Build history of the part. All positions in model axes, mm. A direction names the side the tool comes from. Give positions to 0.01 mm unless a question says otherwise; leave off trailing zeros. Loops run counter-clockwise (first coordinate to the right, second up) from the corner with the lowest first, then second, coordinate; pieces in that order, holes last. Notation, with made-up numbers: (0.25, 17.25) -> (46.25, 17.25) arc R28 ccw to (46.25, 54.25) -> close; hole circle Ø10 at (12, 24.5). An arc over 180 degrees is marked (long way). Answer as a JSON object with one key per item and string values. Group by question number.
Q1. Band-saw the part on A-A, the plane z = 1.4. Write the cut outline in (x, y), plus the area to 3 significant figures.
Q2. Band-saw the part on C-C, the plane y = 53. Write the cut outline in (x, z), plus the area to 3 significant figures.
Q3. Two-plate mould, pull along X, no slides. Class faces 1 (the flat face through (130, 59, 0)), 2 (the cylindrical face through (68.987, 74.602, 1.014)), 3 (the cylindrical face through (131.93, 70.72, 1.51)): pulls with the +X half, pulls with the -X half, needs draft (parallel to the pull), parting line crosses it, or undercut.
Q4. Tool access for faces 4 (the flat face through (127, 71, 1)), 5 (the cylindrical face through (126.93, 72.05, 0.51)): list every direction of +Z, -Z, +X, -X, +Y, -Y with a clear straight run to the whole face (end or side of a thin tool).
Q5. Drop a flat-ended pin along its axis: pin 1 (6 mm diameter, centred on x = 128.93, y = 71.96, fed in from -Z). Give the stop position or say it passes through.
Q6. Wall check: probe 1 along Y at (x, z) = (128.5, 0.8); probe 2 along X at (y, z) = (35, 1.55); probe 3 along Y at (x, z) = (175.5, 1). Give the ranges that are in metal, low to high. Write a range as from..to.
Q7. Band-saw the part on B-B, the plane x = 103. Write the cut outline in (y, z).
Solid Edge part; units mm, degrees
sketch "Sketch1" plane through (0, 0, 0) normal (0, 0, 1) x (1, 0, 0)
  line L0 (68.9286, 131.9643) -> (188.9286, 131.9643)
  line L1 (188.9286, 131.9643) -> (188.9286, 11.9643)
  line L2 (188.9286, 11.9643) -> (68.9286, 11.9643)
  line L3 (68.9286, 11.9643) -> (68.9286, 131.9643)
  dimension "D1" = 68.9286
  dimension "D2" = 188.9286
  dimension "D3" = 68.9286
extrude "Protrusion1" add sketch "Sketch1" along normal blind 2
sketch "Sketch2" plane through (128.9286, 71.9643, 2) normal (0, 0, 1) x (1, 0, 0)
  circle A0 centre (0, 0) radius 2
extrude "Cutout1" cut sketch "Sketch2" against normal through all
sketch "Sketch3" plane through (128.9286, 71.9643, 2) normal (0, 0, 1) x (1, 0, 0)
  circle A0 centre (0, 0) radius 3.25
extrude "ExtrudedCutout_3" cut sketch "Sketch3" against normal blind 1
sketch "Sketch4" plane through (128.9286, 71.9643, 2) normal (0, 0, 1) x (1, 0, 0)
  circle A0 centre (0, 0) radius 60
  circle A1 centre (0, 0) radius 90
extrude "Cutout2" cut sketch "Sketch4" against normal through all
Worked answers:
{
 "1": {"outline": "circle Ø120 at (128.93, 71.96); hole circle Ø6.5 at (128.93, 71.96)", "area": "11,300 mm2"},
 "2": {"outline": "(72, 0) -> (185.85, 0) -> (185.85, 2) -> (72, 2) -> close", "area": "228 mm2"},
 "3": {"face 1": "needs draft", "face 2": "parting line crosses it", "face 3": "undercut"},
 "4": {"face 4": "+Z", "face 5": "+Z, -Z"},
 "5": {"pin 1": "z = 0"},
 "6": {"probe 1": "11.97..70.01, 73.92..131.96", "probe 2": "81.67..176.19", "probe 3": "34.13..109.79"},
 "7": {"outline": "(17.86, 0) -> (126.07, 0) -> (126.07, 2) -> (17.86, 2) -> close"}
}
